from build123d import *

# Parameters (mm, degrees)
SKETCH1_W           = 35
SKETCH1_H           = 40
BOSS_EXTRUDE1_DEPTH = 7
CUT_EXTRUDE1_DEPTH  = 8
FILLET1_R           = 10


with BuildPart() as part:
    # Sketch1 → Boss-Extrude1 (new body)
    with BuildSketch(Plane(origin=(0, 0, 0), x_dir=(1, 0, 0), z_dir=(0, 1, 0))):
        Rectangle(SKETCH1_W, SKETCH1_H)
    extrude(amount=BOSS_EXTRUDE1_DEPTH)

    # Sketch2 → Cut-Extrude1 (cut)
    with BuildSketch(Plane(origin=(0, 7, 0), x_dir=(1, 0, 0), z_dir=(0, 1, 0))):
        with BuildLine():
            Line((15.25007819, 6.222406887), (17.5, 5.083636977))
            Line((17.5, 5.083636977), (17.5, 20))
            Line((17.5, 20), (12.452367732, 5.078850678))
            ThreePointArc((12.452367732, 5.078850678), (13.590179491, 6.289271676), (15.25007819, 6.222406887))
        make_face()
        with BuildLine():
            Line((17.5, -4.742517197), (17.5, 5.083636977))
            Line((17.5, 5.083636977), (15.25007819, 6.222406887))
            ThreePointArc((15.25007819, 6.222406887), (13.590179491, 6.289271676), (12.452367732, 5.078850678))
            ThreePointArc((12.452367732, 5.078850678), (12.374244311, 4.767544782), (12.346923988, 4.447750739))
            Line((12.346923988, 4.447750739), (12.305154889, -4.080011014))
            ThreePointArc((12.305154889, -4.080011014), (12.330174144, -4.405315746), (12.407751507, -4.722224068))
            ThreePointArc((12.407751507, -4.722224068), (13.535222521, -5.935678289), (15.190785632, -5.883020714))
            Line((15.190785632, -5.883020714), (17.5, -4.742517197))
        make_face()
        with BuildLine():
            Line((17.5, -20), (17.5, -4.742517197))
            Line((17.5, -4.742517197), (15.190785632, -5.883020714))
            ThreePointArc((15.190785632, -5.883020714), (13.535222521, -5.935678289), (12.407751507, -4.722224068))
            Line((12.407751507, -4.722224068), (17.5, -20))
        make_face()
        with BuildLine():
            Line((1.11774743, -1.361450371), (6.099320122, -5.135895168))
            ThreePointArc((6.099320122, -5.135895168), (8.192797189, -5.335005696), (9.307118466, -3.551587818))
            Line((9.307118466, -3.551587818), (9.343853133, 3.94832222))
            ThreePointArc((9.343853133, 3.94832222), (8.247055315, 5.742570191), (6.151728246, 5.563976485))
            Line((6.151728246, 5.563976485), (1.133420888, 1.838511245))
            ThreePointArc((1.133420888, 1.838511245), (0.325593755, 0.242448801), (1.11774743, -1.361450371))
        make_face()
        with BuildLine():
            Line((-2.632460294, 8.813664358), (-2.648655993, 5.507079694))
            ThreePointArc((-2.648655993, 5.507079694), (-1.551858174, 3.712831723), (0.543468894, 3.891425428))
            Line((0.543468894, 3.891425428), (5.773694974, 7.774213801))
            ThreePointArc((5.773694974, 7.774213801), (6.574320559, 9.549924863), (5.484724289, 11.164524215))
            Line((5.484724289, 11.164524215), (3.228851981, 12.306305896))
            ThreePointArc((3.228851981, 12.306305896), (2.037191792, 12.574954754), (0.86049862, 12.246900805))
            Line((0.86049862, 12.246900805), (-1.371870903, 10.972579453))
            ThreePointArc((-1.371870903, 10.972579453), (-2.291405376, 10.06200886), (-2.632460294, 8.813664358))
        make_face()
        with BuildLine():
            Line((0.507713818, -3.408487008), (5.699653959, -7.3423233))
            ThreePointArc((5.699653959, -7.3423233), (6.482846631, -9.125791927), (5.377486357, -10.729640351))
            Line((5.377486357, -10.729640351), (3.110537628, -11.849269189))
            ThreePointArc((3.110537628, -11.849269189), (1.916302986, -12.1062319), (0.742879821, -11.766667047))
            Line((0.742879821, -11.766667047), (-1.476899604, -10.470539006))
            ThreePointArc((-1.476899604, -10.470539006), (-2.387470197, -9.551004532), (-2.716280225, -8.299379022))
            Line((-2.716280225, -8.299379022), (-2.700084526, -4.992794358))
            ThreePointArc((-2.700084526, -4.992794358), (-1.585763249, -3.20937648), (0.507713818, -3.408487008))
        make_face()
    extrude(amount=-CUT_EXTRUDE1_DEPTH, mode=Mode.SUBTRACT)

    # Fillet1
    fillet1_edges = [part.edges().sort_by_distance(p)[0] for p in [
        (17.5, 3.5, 20),
        (-17.5, 3.5, 20),
        (-17.5, 3.5, -20),
        (17.5, 3.5, -20),
    ]]
    fillet(fillet1_edges, radius=FILLET1_R)


solid = part.part
Geometry: final body of the model. Coordinates: model frame, mm. A direction names the side the tool comes from. Coordinates: 2 decimals unless noted, no trailing zeros. Write each loop counter-clockwise with the first axis right and the second up, starting at its lowest first coordinate (ties: lowest second). Pieces come first, ordered by that corner, then holes. Notation, with made-up numbers: (86, 17) - (139, 17) arc R9 ccw to (139, 22) - close; hole circle Ø5 at (15.25, 43). An arc over 180 degrees is marked (long way). Return JSON: item names as keys, results as strings.
Item 1: Reachability of faces 4 (the face through (-2.28, 3.55, -10.08)), 5 (the face through (-2, 3, -20)), 6 (the face through (12.747, 3.549, -5.949)) from +Z, -Z, +X, -X, +Y, -Y: full face, straight path, thin tool, end or side. Return the list, or none.
Completed:
{"face 4": "+Y, -Y", "face 5": "-Z, +X, -X, +Y, -Y", "face 6": "+X, +Y, -Y"}
Item 2: Section query B-B (z = 0). Output: boundary loops of the cut face in (x, y), and give its area (3 significant figures).
Completed:
{"outline": "(-17.5, 0) - (0.34, 0) - (0.34, 7) - (-17.5, 7) - close; (9.32, 0) - (12.33, 0) - (12.33, 7) - (9.32, 7) - close", "area": "146 mm2"}
Item 3: Section query C-C (x = 2). Output: boundary loops of the cut face in (y, z), and give its area (3 significant figures).
Completed:
{"outline": "(0, -20) - (7, -20) - (7, -12.57) - (0, -12.57) - close; (0, -4.97) - (7, -4.97) - (7, -2.48) - (0, -2.48) - close; (0, 2.03) - (7, 2.03) - (7, 4.54) - (0, 4.54) - close; (0, 12.11) - (7, 12.11) - (7, 20) - (0, 20) - close", "area": "142 mm2"}
Item 4: Section query A-A (y = 0.5). Count the separate pieces of the cut face and the enclosed holes in it, and give its area (3 significant figures).
Completed:
{"separate pieces": "1", "enclosed holes": "3", "area": "955 mm2"}
Item 5: Line query: L1, parallel to Z at x = 3, y = 2.5; L2, parallel to X at y = 3, z = -11.5; L3, parallel to Z at x = -1, y = 6.25. Output: solid intervals per line, ascending.
Completed:
{"L1": "z = -20 to -12.41, -5.72 to -3.22, 2.79 to 5.3, 11.9 to 20", "L2": "x = -17.39 to -0.45, 4.82 to 13.45", "L3": "z = -20 to -11.18, -3.53 to 3.03, 10.75 to 20"}
Item 6: Section query D-D (x = -13.5). Output: boundary loops of the cut face in (y, z), and give its area (3 significant figures).
Completed:
{"outline": "(0, -18) - (7, -18) - (7, 18) - (0, 18) - close", "area": "252 mm2"}
Item 7: Pull-direction query (X, two-part tool) for faces 1 (the face through (3.122, 3.549, -5.806)), 2 (the face through (-2, 3, 20)), 3 (the face through (-14.65, 3.55, -16.99)); classes: +X half, -X half, draft (parallel to the pull), parting line (faces both ways), or undercut.
Completed:
{"face 1": "undercut", "face 2": "draft", "face 3": "-X half"}
